```python
from build123d import *

# Parameters (mm, degrees)
SKETCH001_W     = 25.4
SKETCH001_H     = 25.4
PAD001_DEPTH    = 609.6
SKETCH002_R     = 8.89
SKETCH002_R_2   = 1.6
POCKET_DEPTH    = 5.08
SKETCH003_R     = 4
POCKET001_DEPTH = 25.401
POCKET002_DEPTH = 25.401
POCKET006_DEPTH = 25.401
PAD004_DEPTH    = 19.05
SKETCH020_R     = 3.302
POCKET012_DEPTH = 7.62
SKETCH021_R     = 3.175
POCKET013_DEPTH = 22.226


with BuildPart() as part:
    # Sketch001 → Pad001 (new body)
    with BuildSketch(Plane.XY):
        Rectangle(SKETCH001_W, SKETCH001_H)
        with BuildLine():
            ThreePointArc((-9.525, -6.35), (-8.595064, -8.595064), (-6.35, -9.525))
            Line((6.35, -9.525), (-6.35, -9.525))
            ThreePointArc((6.35, -9.525), (8.595064, -8.595064), (9.525, -6.35))
            Line((9.525, 6.35), (9.525, -6.35))
            ThreePointArc((9.525, 6.35), (8.595064, 8.595064), (6.35, 9.525))
            Line((-6.35, 9.525), (6.35, 9.525))
            ThreePointArc((-6.35, 9.525), (-8.595064, 8.595064), (-9.525, 6.35))
            Line((-9.525, -6.35), (-9.525, 6.35))
        make_face(mode=Mode.SUBTRACT)
    extrude(amount=PAD001_DEPTH)

    # Sketch002 (on Face2 of Pad001) → Pocket (cut)
    with BuildSketch(Plane(origin=(0, 12.7, 0), x_dir=(-1, 0, 0), z_dir=(0, 1, 0))):
        with Locations((0, 558.8)):
            Circle(SKETCH002_R)
        with Locations((0, 580.72031)):
            Circle(SKETCH002_R_2)
        with Locations((0, 536.87969)):
            Circle(SKETCH002_R_2)
    extrude(amount=-POCKET_DEPTH, mode=Mode.SUBTRACT)

    # Sketch003 (on Face1 of Pocket) → Pocket001 (cut, through all)
    with BuildSketch(Plane(origin=(-12.7, 0, 0), x_dir=(0, -1, 0), z_dir=(-1, 0, 0))):
        with Locations((0, 584.2)):
            Circle(SKETCH003_R)
        with Locations((0, 533.4)):
            Circle(SKETCH003_R)
    extrude(amount=-POCKET001_DEPTH, mode=Mode.SUBTRACT)

    # Sketch004 (on Face2 of Pocket001) → Pocket002 (cut, through all)
    with BuildSketch(Plane.XZ.offset(12.7)):
        Polygon((12.7, 0), (-12.7, 0), (-12.7, 25.4), align=None)
    extrude(amount=-POCKET002_DEPTH, mode=Mode.SUBTRACT)

    # Sketch010 (on Face8 of Pocket002) → Pocket006 (cut, through all)
    with BuildSketch(Plane.YZ.offset(12.7)):
        with BuildLine():
            ThreePointArc((-7.62, 544.5125), (-6.225096, 541.144904), (-2.8575, 539.75))
            Line((2.8575, 539.75), (-2.8575, 539.75))
            ThreePointArc((2.8575, 539.75), (6.225096, 541.144904), (7.62, 544.5125))
            Line((7.62, 573.0875), (7.62, 544.5125))
            ThreePointArc((7.62, 573.0875), (6.225096, 576.455096), (2.8575, 577.85))
            Line((-2.8575, 577.85), (2.8575, 577.85))
            ThreePointArc((-2.8575, 577.85), (-6.225096, 576.455096), (-7.62, 573.0875))
            Line((-7.62, 544.5125), (-7.62, 573.0875))
        make_face()
    extrude(amount=-POCKET006_DEPTH, mode=Mode.SUBTRACT)

    # Sketch014 (on DatumPlane) → Pad004 (join)
    with BuildSketch(Plane(origin=(-9.525, 0, 0), x_dir=(0, -1, 0), z_dir=(-1, 0, 0))):
        Polygon((12.7, 31.75), (12.7, 64.962661), (50.536436, 10.926631), (34.931589, 0), align=None)
        Polygon((-12.7, 64.962661), (-12.7, 31.75), (-34.931589, 0), (-50.536436, 10.926631), align=None)
    extrude(amount=-PAD004_DEPTH)

    # Sketch020 (on Face3 of Pad004) → Pocket012 (cut)
    with BuildSketch(Plane.XZ.offset(12.7)):
        with Locations((0, 536.87969)):
            Circle(SKETCH020_R)
        with Locations((0, 580.72031)):
            Circle(SKETCH020_R)
    extrude(amount=-POCKET012_DEPTH, mode=Mode.SUBTRACT)

    # Sketch021 (on Face29 of Pocket012) → Pocket013 (cut, through all)
    with BuildSketch(Plane.YZ.offset(9.525)):
        with Locations((-28.165171, 26.269777)):
            Circle(SKETCH021_R)
        with Locations((28.165171, 26.269777)):
            Circle(SKETCH021_R)
    extrude(amount=-POCKET013_DEPTH, mode=Mode.SUBTRACT)


solid = part.part
```
The model under review builds one solid part; all positions refer to its coordinate system, in mm. A direction names the side the tool comes from. Round coordinates to 2 decimals unless told otherwise and drop trailing zeros. Write each loop counter-clockwise with the first axis right and the second up, starting at its lowest first coordinate (ties: lowest second). Pieces come first, ordered by that corner, then holes.
(1) Machinability: for faces 1 (the flat face through (9.525, -32, 26)), 2 (the flat face through (-0.2, -11.5, 12.9)), 3 (the flat face through (0, -9.525, 304)), which of the approach directions +Z, -Z, +X, -X, +Y, -Y give a long, thin tool a straight path to every point of the face, cutting with its end or side? Answer none if there is none.
(2) We need section A-A on z = 558.8. Give the boundary of the cut face in (x, y) (3 decimals).
(3) We need section B-B on z = 416. Give the boundary of the cut face in (x, y) (3 decimals), and give its area (3 significant figures).
(4) We need section C-C on y = 40. Give the boundary of the cut face in (x, z) (3 decimals), and give its area (3 significant figures).
(5) Mouldability with a two-part tool opening along Z and no side actions: class faces 4 (the flat face through (0, 11, 609.6)), 5 (the cylindrical face through (8.88, 11, 559.19)), 6 (the flat face through (-9.525, 0, 593)) as +Z half, -Z half, draft (parallel to the pull), parting line (faces both ways), or undercut.
(6) We need section D-D on y = -18.5. Give the boundary of the cut face in (x, z) (3 decimals).
(7) Insertion check: pin 1 (1.7 mm diameter, centred on x = 10.5, z = 564.5, fed in from +Y); pin 2 (19 mm diameter, centred on y = -28, z = 45.5, fed in from -X) (3 decimals); pin 3 (10 mm diameter, centred on x = 1.5, z = 229.5, fed in from -Y). Each pin has a flat end and moves straight along its axis. Give the tip position at first contact, or say it passes through.
(8) Wall thickness on L1, parallel to Y at x = -3.5, z = 143.5 (3 decimals); L2, parallel to Y at x = -10.6, z = 584.2: over which ranges is each line inside the solid? List them lowest first.
Findings below:
1. face 1: +Z, -Z, +X, -Y
1. face 2: -Z, -X
1. face 3: +Z, -Z
2. outline: (-12.7, -12.7) - (12.7, -12.7) - (12.7, -7.62) - (9.26, -7.62) arc R3.175 cw to (6.35, -9.525) - (-6.35, -9.525) arc R3.175 cw to (-9.26, -7.62) - (-12.7, -7.62) - close; (-12.7, 7.62) - (-9.26, 7.62) arc R3.175 cw to (-8.89, 8.255) - (-8.89, 12.7) - (-12.7, 12.7) - close; (8.89, 8.255) arc R3.175 cw to (9.26, 7.62) - (12.7, 7.62) - (12.7, 12.7) - (8.89, 12.7) - close
3. outline: (-12.7, -12.7) - (12.7, -12.7) - (12.7, 12.7) - (-12.7, 12.7) - close; hole (-9.525, -6.35) arc R3.175 ccw to (-6.35, -9.525) - (6.35, -9.525) arc R3.175 ccw to (9.525, -6.35) - (9.525, 6.35) arc R3.175 ccw to (6.35, 9.525) - (-6.35, 9.525) arc R3.175 ccw to (-9.525, 6.35) - close
3. area: 291 mm2
4. outline: (-9.525, 3.549) - (9.525, 3.549) - (9.525, 25.974) - (-9.525, 25.974) - close
4. area: 427 mm2
5. face 4: +Z half
5. face 5: undercut
5. face 6: draft
6. outline: (-9.525, 23.467) - (9.525, 23.467) - (9.525, 56.679) - (-9.525, 56.679) - close
7. pin 1: stops at y = 12.7
7. pin 2: stops at x = -9.525
7. pin 3: stops at y = -12.7
8. L1: y = -12.7 to -9.525, 9.525 to 12.7
8. L2: y = -12.7 to -4, 4 to 12.7
